Verification items for the finished model (mm, model axes). Round coordinates to 2 decimals unless told otherwise and drop trailing zeros. Write each loop counter-clockwise with the first axis right and the second up, starting at its lowest first coordinate (ties: lowest second). Pieces come first, ordered by that corner, then holes. Notation, with made-up numbers: M 8,14.5 L 51,14.5 A17 cw 51,46.5 Z; hole C -28.75,11.25 d1. An arc over 180 degrees is marked long. One line per question, with ' | ' between items.
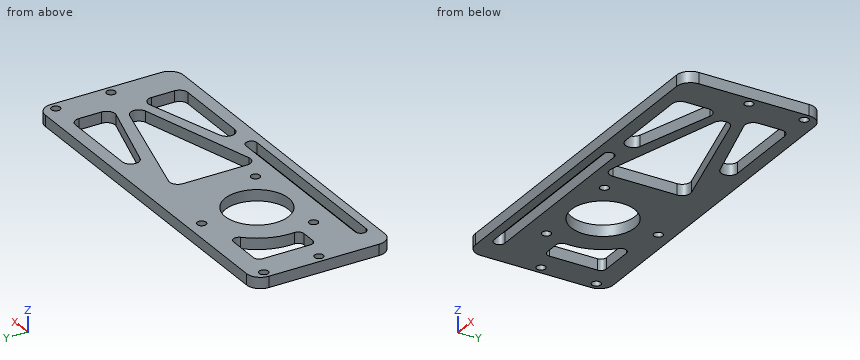
from build123d import *

# Parameters (mm, degrees)
SKETCH_1_W          = 130
SKETCH_1_H          = 50
SKETCH_1_R          = 11.5
SKETCH_1_R_2        = 1.6
EXTRUDE_1_DEPTH     = 2
SKETCH_2_R          = 1.6
CUT_EXTRUDE_1_DEPTH = 70.756720106
FILLET_1_R          = 5
CUT_EXTRUDE_2_DEPTH = 70.756720106
FILLET_2_R          = 3
CUT_EXTRUDE_3_DEPTH = 70.756720106
FILLET_3_R          = 2


with BuildPart() as part:
    # 草图1 → 凸台-拉伸1 (new, symmetric)
    with BuildSketch(Plane.XY):
        Rectangle(SKETCH_1_W, SKETCH_1_H)
        with Locations((-25, 0)):
            Circle(SKETCH_1_R, mode=Mode.SUBTRACT)
        with Locations((-25, 20)):
            Circle(SKETCH_1_R_2, mode=Mode.SUBTRACT)
        with Locations((-7.679491924, -10)):
            Circle(SKETCH_1_R_2, mode=Mode.SUBTRACT)
        with Locations((-42.320508076, -10)):
            Circle(SKETCH_1_R_2, mode=Mode.SUBTRACT)
    extrude(amount=EXTRUDE_1_DEPTH, both=True)

    # 草图2 → 切除-拉伸1 (cut, through all)
    with BuildSketch(Plane.XY.offset(2)):
        with Locations((-62, 0)):
            Circle(SKETCH_2_R)
        with Locations((-62, 20)):
            Circle(SKETCH_2_R)
        with Locations(Location((62, 0, 0), (0, 0, 180))):
            Circle(SKETCH_2_R)
        with Locations(Location((62, 20, 0), (0, 0, 180))):
            Circle(SKETCH_2_R)
    extrude(amount=-CUT_EXTRUDE_1_DEPTH, mode=Mode.SUBTRACT)

    # 圆角1
    fillet_1_edges = [part.edges().sort_by_distance(p)[0] for p in [
        (65, -25, 0),
        (-65, -25, 0),
        (-65, 25, 0),
        (65, 25, 0),
    ]]
    fillet(fillet_1_edges, radius=FILLET_1_R)

    # 草图3 → 切除-拉伸2 (cut, through all)
    with BuildSketch(Plane.XY.offset(2)):
        Polygon((0, -15.574230951), (0, 15.574230951), (56.674910039, 0), align=None)
        Polygon((52.704928418, -20.329043818), (1.183129779, -20.329043818), (52.704928418, -4.996701006), align=None)
        Polygon((1.183129779, 20.329043818), (52.704928418, 4.996701006), (52.704928418, 20.329043818), align=None)
    extrude(amount=-CUT_EXTRUDE_2_DEPTH, mode=Mode.SUBTRACT)

    # 圆角2
    fillet_2_edges = [part.edges().sort_by_distance(p)[0] for p in [
        (1.183129779, 20.329043818, 0),
        (52.704928418, 20.329043818, 0),
        (52.704928418, 4.996701006, 0),
        (52.704928418, -4.996701006, 0),
        (52.704928418, -20.329043818, 0),
        (1.183129779, -20.329043818, 0),
        (56.674910039, 0, 0),
        (0, -15.574230951, 0),
        (0, 15.574230951, 0),
    ]]
    fillet(fillet_2_edges, radius=FILLET_2_R)

    # 草图4 → 切除-拉伸3 (cut, through all)
    with BuildSketch(Plane.XY.offset(2)):
        with BuildLine():
            Line((-34.180193003, 17.76862562), (-54.308419113, 17.76862562))
            Line((-54.308419113, 17.76862562), (-54.308419113, -3.656277433))
            Line((-54.308419113, -3.656277433), (-44.66295083, -3.656277433))
            ThreePointArc((-44.66295083, -3.656277433), (-42.964920101, 8.789860395), (-34.180193003, 17.76862562))
        make_face()
        with BuildLine():
            Line((-54.308419113, -17.77082873), (10.857927113, -17.77082873))
            ThreePointArc((10.857927113, -17.77082873), (12.857927113, -19.77082873), (10.857927113, -21.77082873))
            Line((10.857927113, -21.77082873), (-54.308419113, -21.77082873))
            ThreePointArc((-54.308419113, -21.77082873), (-56.308419113, -19.77082873), (-54.308419113, -17.77082873))
        make_face()
    extrude(amount=-CUT_EXTRUDE_3_DEPTH, mode=Mode.SUBTRACT)

    # 圆角3
    fillet_3_edges = [part.edges().sort_by_distance(p)[0] for p in [
        (-34.180193003, 17.76862562, 0),
        (-44.66295083, -3.656277433, 0),
        (-54.308419113, -3.656277433, 0),
        (-54.308419113, 17.76862562, 0),
    ]]
    fillet(fillet_3_edges, radius=FILLET_3_R)


solid = part.part
1. Go/stop test with a flat-tipped pin: P1, Ø14, axis at x = -25, y = 0, coming from the +Z side. Record where the tip stops, or that it passes through.
Results:
P1: passes through
2. Section check C-C, the plane y = 7.5. Record the cut outline in (x, z), then the cut area to 3 significant figures.
Results:
outline: M -65,-2 L -54.31,-2 L -54.31,2 L -65,2 Z; M -43.54,-2 L -33.72,-2 L -33.72,2 L -43.54,2 Z; M -16.28,-2 L 0,-2 L 0,2 L -16.28,2 Z; M 29.38,-2 L 44.29,-2 L 44.29,2 L 29.38,2 Z; M 52.29,-2 L 65,-2 L 65,2 L 52.29,2 Z | area: 258 mm2
3. Section check D-D, the plane x = 26.5. Record the cut outline in (y, z), then the cut area to 3 significant figures.
Results:
outline: M -25,-2 L -20.33,-2 L -20.33,2 L -25,2 Z; M -12.8,-2 L -8.29,-2 L -8.29,2 L -12.8,2 Z; M 8.29,-2 L 12.8,-2 L 12.8,2 L 8.29,2 Z; M 20.33,-2 L 25,-2 L 25,2 L 20.33,2 Z | area: 73.4 mm2
4. Thickness scan on line 1 (Y direction, x = -25, z = 0); line 2 (Y direction, x = -35, z = -1.35); line 3 (X direction, y = 16, z = 1.75) (1 decimal). Record the ranges inside material, lowest first.
Results:
line 1: y = -25 to -21.77, -17.77 to -11.5, 11.5 to 18.4, 21.6 to 25 | line 2: y = -25 to -21.77, -17.77 to -5.68, 5.68 to 25 | line 3: x = -65 to -54.3, -38.4 to 19.1, 52.7 to 65
5. Section check A-A, the plane y = 0. Record the cut outline in (x, z).
Results:
outline: M -65,-2 L -63.6,-2 L -63.6,2 L -65,2 Z; M -60.4,-2 L -54.31,-2 L -54.31,2 L -60.4,2 Z; M -45,-2 L -36.5,-2 L -36.5,2 L -45,2 Z; M -13.5,-2 L 0,-2 L 0,2 L -13.5,2 Z; M 48.35,-2 L 60.4,-2 L 60.4,2 L 48.35,2 Z; M 63.6,-2 L 65,-2 L 65,2 L 63.6,2 Z
6. Section check B-B, the plane x = 1.5. Record the cut outline in (y, z), then the cut area to 3 significant figures.
Results:
outline: M -25,-2 L -21.77,-2 L -21.77,2 L -25,2 Z; M -17.77,-2 L -14.24,-2 L -14.24,2 L -17.77,2 Z; M 14.24,-2 L 25,-2 L 25,2 L 14.24,2 Z | area: 70.1 mm2
